from build123d import *

# Parameters (mm, degrees)
CROQUIS1_R              = 40
CROQUIS1_R_2            = 12.5
SALIENTE_EXTRUIR1_DEPTH = 10


with BuildPart() as part:
    # Croquis1 → Saliente-Extruir1 (new body)
    with BuildSketch(Plane.XY):
        with BuildLine():
            ThreePointArc((79.950643702, 2.809728022), (24.958439712, 76.007080507), (-62.721500941, 49.658970184))
            ThreePointArc((-62.721500941, 49.658970184), (-24.43428434, -137.747119815), (153.67978893, -68.016707318))
            ThreePointArc((153.67978893, -68.016707318), (149.121265752, -43.894808413), (126.125371367, -35.302079987))
            ThreePointArc((126.125371367, -35.302079987), (94.463628593, -26.634547282), (79.950643702, 2.809728022))
        make_face()
        Circle(CROQUIS1_R, mode=Mode.SUBTRACT)
        with Locations((130, -60)):
            Circle(CROQUIS1_R_2, mode=Mode.SUBTRACT)
        with Locations((99.358222275, -85.711504387)):
            Circle(CROQUIS1_R_2, mode=Mode.SUBTRACT)
        with Locations((68.71644455, -111.423008775)):
            Circle(CROQUIS1_R_2, mode=Mode.SUBTRACT)
        with Locations((38.074666826, -137.134513162)):
            Circle(CROQUIS1_R_2, mode=Mode.SUBTRACT)
        with Locations((80.074593985, -62.730171094)):
            Circle(CROQUIS1_R_2, mode=Mode.SUBTRACT)
        with Locations((49.43281626, -88.441675481)):
            Circle(CROQUIS1_R_2, mode=Mode.SUBTRACT)
        with Locations((18.791038535, -114.153179869)):
            Circle(CROQUIS1_R_2, mode=Mode.SUBTRACT)
        with Locations((30.149187969, -65.460342188)):
            Circle(CROQUIS1_R_2, mode=Mode.SUBTRACT)
        with Locations((-0.492589755, -91.171846575)):
            Circle(CROQUIS1_R_2, mode=Mode.SUBTRACT)
        with Locations((-19.776218046, -68.190513282)):
            Circle(CROQUIS1_R_2, mode=Mode.SUBTRACT)
    extrude(amount=SALIENTE_EXTRUIR1_DEPTH)


solid = part.part
Work out the finished part from the listing and answer in its coordinate system (mm). Coordinates: 2 decimals unless noted, no trailing zeros. Write each loop counter-clockwise with the first axis right and the second up, starting at its lowest first coordinate (ties: lowest second). Pieces come first, ordered by that corner, then holes.
1. The part is cut by section B-B, the plane y = 17.5. Write down the section's boundary in (x, z).
Results list:
outline: (-81.17, 0) - (-35.97, 0) - (-35.97, 10) - (-81.17, 10) - close; (35.97, 0) - (78.06, 0) - (78.06, 10) - (35.97, 10) - close
2. The part is cut by section A-A, the plane x = 130. Write down the section's boundary in (y, z).
Results list:
outline: (-109.5, 0) - (-72.5, 0) - (-72.5, 10) - (-109.5, 10) - close; (-47.5, 0) - (-35, 0) - (-35, 10) - (-47.5, 10) - close
3. Consider line 1 along X through (y, z) = (-84, 6.5); line 2 along Y through (x, z) = (89, 2.25); line 3 along Y through (x, z) = (19, 0.5). Determine where each line is inside the solid, lowest interval first.
Results list:
line 1: x = -76.44 to -10.73, 9.75 to 37.75, 61.12 to 86.98, 111.74 to 147
line 2: y = -140.8 to -92.71, -78.71 to -71.48, -53.98 to -21.15
line 3: y = -151.87 to -126.65, -101.65 to -71.11, -59.81 to -35.2, 35.2 to 77.71
4. For a pull along Y with two mould halves and no side action, classify faces 1 (the cylindrical face through (26.25, 75.57, 4.93)), 2 (the cylindrical face through (-2.12, -78.78, 4.93)), 3 (the flat face through (31, -35, 0)) as +Y half, -Y half, draft (parallel to the pull), parting line (faces both ways), or undercut.
Results list:
face 1: +Y half
face 2: undercut
face 3: draft
5. The part is cut by section D-D, the plane x = 9. Write down the section's boundary in (y, z).
Results list:
outline: (-150.14, 0) - (-121.92, 0) - (-121.92, 10) - (-150.14, 10) - close; (-106.38, 0) - (-99.3, 0) - (-99.3, 10) - (-106.38, 10) - close; (-83.04, 0) - (-38.97, 0) - (-38.97, 10) - (-83.04, 10) - close; (38.97, 0) - (79.49, 0) - (79.49, 10) - (38.97, 10) - close
6. The part is cut by section C-C, the plane z = 1.75. State how many separate pieces and enclosed holes the cut face has, and give its area (3 significant figures).
Results list:
separate pieces: 1
enclosed holes: 11
area: 29,000 mm2
7. Flat-ended cylindrical pins translate along their axes: pin 1 (4 mm diameter, centred on x = 128, z = 2, fed in from +Y); pin 2 (5 mm diameter, centred on y = -77, z = 7.5, fed in from -X); pin 3 (5 mm diameter, centred on y = -47, z = 4.5, fed in from -X). Find the tip coordinate at first contact, or state that the pin passes through.
Results list:
pin 1: stops at y = -35
pin 2: stops at x = -80.72
pin 3: stops at x = -88.62
